```python
from build123d import *

# Parameters (mm, degrees)
SKETCH_1_W          = 91
SKETCH_1_H          = 50
SKETCH_1_W_2        = 83
SKETCH_1_H_2        = 36
EXTRUDE_1_DEPTH     = 3
SKETCH_2_R          = 1.5
CUT_EXTRUDE_1_DEPTH = 3
SKETCH_3_R          = 1.6
CUT_EXTRUDE_2_DEPTH = 3
FILLET_1_R          = 4
SKETCH_4_W          = 30
SKETCH_4_H          = 35
EXTRUDE_2_DEPTH     = 3
SKETCH_5_R          = 1.25
CUT_EXTRUDE_3_DEPTH = 10
FILLET_2_R          = 3
SKETCH_6_W          = 18
SKETCH_6_H          = 27
CUT_EXTRUDE_4_DEPTH = 10
FILLET_3_R          = 2
SKETCH_7_W          = 38
SKETCH_7_H          = 10
SKETCH_7_R          = 1.6
EXTRUDE_3_DEPTH     = 3
FILLET_4_R          = 2
FILLET_5_R          = 2
SKETCH_8_W          = 42
SKETCH_8_H          = 10
CUT_EXTRUDE_5_DEPTH = 10


with BuildPart() as part:
    # 草图1 → 凸台-拉伸1 (new body)
    with BuildSketch(Plane.XY):
        Rectangle(SKETCH_1_W, SKETCH_1_H)
        Rectangle(SKETCH_1_W_2, SKETCH_1_H_2, mode=Mode.SUBTRACT)
    extrude(amount=EXTRUDE_1_DEPTH)

    # 草图2 → 切除-拉伸1 (cut)
    with BuildSketch(Plane.XY.offset(3)):
        with Locations((31.5, 21)):
            Circle(SKETCH_2_R)
        with Locations((31.5, -21)):
            Circle(SKETCH_2_R)
        with Locations((-31.5, -21)):
            Circle(SKETCH_2_R)
        with Locations((-31.5, 21)):
            Circle(SKETCH_2_R)
    extrude(amount=-CUT_EXTRUDE_1_DEPTH, mode=Mode.SUBTRACT)

    # 草图3 → 切除-拉伸2 (cut)
    with BuildSketch(Plane.XY.offset(3)):
        with Locations((41.5, 20)):
            Circle(SKETCH_3_R)
        with Locations((41.5, -20)):
            Circle(SKETCH_3_R)
        with Locations((-41.5, -20)):
            Circle(SKETCH_3_R)
        with Locations((-41.5, 20)):
            Circle(SKETCH_3_R)
    extrude(amount=-CUT_EXTRUDE_2_DEPTH, mode=Mode.SUBTRACT)

    # 圆角1
    fillet_1_edges = [part.edges().sort_by_distance(p)[0] for p in [
        (41.5, -18, 1.5),
        (41.5, 18, 1.5),
        (-41.5, 18, 1.5),
        (-41.5, -18, 1.5),
        (45.5, -25, 1.5),
        (-45.5, -25, 1.5),
        (-45.5, 25, 1.5),
        (45.5, 25, 1.5),
    ]]
    fillet(fillet_1_edges, radius=FILLET_1_R)

    # 草图4 → 凸台-拉伸2 (add)
    with BuildSketch(Plane(origin=(0, 0, 0), x_dir=(-1, 0, 0), z_dir=(0, 0, -1))):
        with Locations((-60.5, 0)):
            Rectangle(SKETCH_4_W, SKETCH_4_H)
    extrude(amount=-EXTRUDE_2_DEPTH)

    # 草图5 → 切除-拉伸3 (cut)
    with BuildSketch(Plane(origin=(0, 0, 0), x_dir=(-1, 0, 0), z_dir=(0, 0, -1))):
        with Locations((-70.5, -12)):
            Circle(SKETCH_5_R)
        with Locations((-70.5, 12)):
            Circle(SKETCH_5_R)
    extrude(amount=-CUT_EXTRUDE_3_DEPTH, mode=Mode.SUBTRACT)

    # 圆角2
    fillet_2_edges = [part.edges().sort_by_distance(p)[0] for p in [
        (45.5, 17.5, 1.5),
        (45.5, -17.5, 1.5),
        (75.5, -17.5, 1.5),
        (75.5, 17.5, 1.5),
    ]]
    fillet(fillet_2_edges, radius=FILLET_2_R)

    # 草图6 → 切除-拉伸4 (cut)
    with BuildSketch(Plane(origin=(0, 0, 0), x_dir=(-1, 0, 0), z_dir=(0, 0, -1))):
        with Locations((-57.5, 0)):
            Rectangle(SKETCH_6_W, SKETCH_6_H)
    extrude(amount=-CUT_EXTRUDE_4_DEPTH, mode=Mode.SUBTRACT)

    # 圆角3
    fillet_3_edges = [part.edges().sort_by_distance(p)[0] for p in [
        (66.5, -13.5, 1.5),
        (66.5, 13.5, 1.5),
        (48.5, 13.5, 1.5),
        (48.5, -13.5, 1.5),
    ]]
    fillet(fillet_3_edges, radius=FILLET_3_R)

    # 草图7 → 凸台-拉伸3 (add)
    # profile 1 of 2: a face of its own
    with BuildSketch(Plane(origin=(0, 0, 0), x_dir=(-1, 0, 0), z_dir=(0, 0, -1))):
        with Locations((0, 30)):
            Rectangle(SKETCH_7_W, SKETCH_7_H)
        with Locations((-16, 32)):
            Circle(SKETCH_7_R, mode=Mode.SUBTRACT)
        with Locations((16, 32)):
            Circle(SKETCH_7_R, mode=Mode.SUBTRACT)
    # profile 2 of 2: a face of its own
    with BuildSketch(Plane(origin=(0, 0, 0), x_dir=(-1, 0, 0), z_dir=(0, 0, -1))):
        with Locations((0, -30)):
            Rectangle(SKETCH_7_W, SKETCH_7_H)
        with Locations((16, -32)):
            Circle(SKETCH_7_R, mode=Mode.SUBTRACT)
        with Locations((-16, -32)):
            Circle(SKETCH_7_R, mode=Mode.SUBTRACT)
    extrude(amount=-EXTRUDE_3_DEPTH)

    # 圆角4
    fillet_4_edges = [part.edges().sort_by_distance(p)[0] for p in [
        (19, 35, 1.5),
        (-19, 35, 1.5),
        (-19, -35, 1.5),
        (19, -35, 1.5),
    ]]
    fillet(fillet_4_edges, radius=FILLET_4_R)

    # 圆角5
    fillet_5_edges = [part.edges().sort_by_distance(p)[0] for p in [
        (19, 25, 1.5),
        (-19, 25, 1.5),
        (-19, -25, 1.5),
        (19, -25, 1.5),
    ]]
    fillet(fillet_5_edges, radius=FILLET_5_R)

    # 草图8 → 切除-拉伸5 (cut)
    with BuildSketch(Plane.XY.offset(3)):
        with Locations((0, 30)):
            Rectangle(SKETCH_8_W, SKETCH_8_H)
        with Locations((0, -30)):
            Rectangle(SKETCH_8_W, SKETCH_8_H)
    extrude(amount=-CUT_EXTRUDE_5_DEPTH, mode=Mode.SUBTRACT)


solid = part.part
```
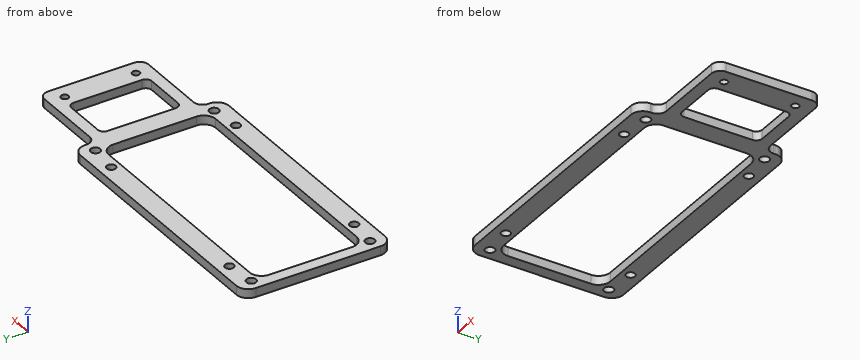
Design review of the part built by this model. Coordinates are the model's own, in mm. Coordinates: 2 decimals unless noted, no trailing zeros. Order: outer loops, then holes, each group sorted by start corner. A loop starts at its lowest first (then second) coordinate and runs counter-clockwise, first axis right, second up. Notation, with made-up numbers: (72, 85.5) - (114, 85.5) arc R30 cw to (114, 113.5) - close; hole circle Ø6 at (44.25, -7.5). An arc over 180 degrees is marked (long way). Answer in a Markdown table with one row per item.
(1) Consider section C-C on x = 31.5. State the section outline as (y, z) points.
Checked values:
| item | result |
|---|---|
| outline | (-25, 0) - (-22.5, 0) - (-22.5, 3) - (-25, 3) - close; (-19.5, 0) - (-18, 0) - (-18, 3) - (-19.5, 3) - close; (18, 0) - (19.5, 0) - (19.5, 3) - (18, 3) - close; (22.5, 0) - (25, 0) - (25, 3) - (22.5, 3) - close |
(2) Consider section A-A on x = 70.5. State the section outline as (y, z) points.
Checked values:
| item | result |
|---|---|
| outline | (-17.5, 0) - (-13.25, 0) - (-13.25, 3) - (-17.5, 3) - close; (-10.75, 0) - (10.75, 0) - (10.75, 3) - (-10.75, 3) - close; (13.25, 0) - (17.5, 0) - (17.5, 3) - (13.25, 3) - close |
(3) Consider section D-D on z = 0.45. Give the number of separate pieces and of enclosed holes in the cut face, plus the area to 3 significant figures.
Checked values:
| item | result |
|---|---|
| separate pieces | 1 |
| enclosed holes | 12 |
| area | 2,060 mm^2 |
(4) Consider section B-B on x = 57.5. State the section outline as (y, z) points.
Checked values:
| item | result |
|---|---|
| outline | (-17.5, 0) - (-13.5, 0) - (-13.5, 3) - (-17.5, 3) - close; (13.5, 0) - (17.5, 0) - (17.5, 3) - (13.5, 3) - close |
(5) Wall thickness on line 1 along X through (y, z) = (-3.5, 2.3); line 2 along Y through (x, z) = (31.5, 2.3); line 3 along Y through (x, z) = (9, 1.75): over which ranges is each line inside the solid? List them lowest first. Write a range as from..to.
Checked values:
| item | result |
|---|---|
| line 1 | -45.5..-41.5, 41.5..48.5, 66.5..75.5 |
| line 2 | -25..-22.5, -19.5..-18, 18..19.5, 22.5..25 |
| line 3 | -25..-18, 18..25 |
(6) Clearance check with flat-ended pins moving along their axes: pin 1 (1.5 mm diameter, centred on x = 59.5, z = 1, fed in from +Y); pin 2 (0.6 mm diameter, centred on y = 20.5, z = 2, fed in from +X); pin 3 (1.9 mm diameter, centred on x = -41.5, y = 20, fed in from -Z); pin 4 (0.9 mm diameter, centred on x = 54.5, z = 1.5, fed in from -Y). State where each tip first meets the part, or that it passes through.
Checked values:
| item | result |
|---|---|
| pin 1 | y = 17.5 |
| pin 2 | x = 45.52 |
| pin 3 | through |
| pin 4 | y = -17.5 |
